Read the model definition and answer for the solid it produces. Units are mm, in the model's axes. A direction names the side the tool comes from. Coordinates: 2 decimals unless noted, no trailing zeros. Write each loop counter-clockwise with the first axis right and the second up, starting at its lowest first coordinate (ties: lowest second). Pieces come first, ordered by that corner, then holes. Notation, with made-up numbers: (-15.75, 87.5) -> (6.25, 87.5) arc R26 ccw to (6.25, 115.5) -> close; hole circle Ø1 at (78.5, 81). An arc over 180 degrees is marked (long way). Answer in a Markdown table with one row per item. Add a question column.
Item 1: Section A-A on y = 16.25 is taken. Write down the section's boundary in (x, z), then the cut area to 3 significant figures.
Item 2: Straight lines are drawn through the part: line 1 (X direction, y = 19, z = -22.1); line 2 (Z direction, x = -20, y = 2.5); line 3 (Z direction, x = 14.5, y = 14). For each, find the intervals that lie inside material, in ascending order. Write a range as from..to.
Item 3: Section D-D on y = 18.75 is taken. Write down the section's boundary in (x, z), then the cut area to 3 significant figures.
Item 4: For a pull along Z with two mould halves and no side action, classify faces 4 (the face through (16, 17, 4)), 5 (the face through (-0.766, 19.788, -20.253)), 6 (the face through (0, 20, -16.1)) as +Z half, -Z half, draft (parallel to the pull), parting line (faces both ways), or undercut.
Item 5: Section C-C on z = -17 is taken. Write down the section's boundary in (x, y).
Item 6: Section B-B on x = 0 is taken. Write down the section's boundary in (y, z).
Item 7: Given pin 1 Ø5 at (x, z) = (-15, -19) entering from -Y; pin 2 Ø3 at (x, y) = (3, 20.5) entering from +Z; pin 3 Ø6 at (x, z) = (-4.5, 1) entering from +Y; pin 4 Ø1.5 at (y, z) = (16.5, -0.5) entering from -X, each flat-ended and moving along its own axis, determine where each tip first touches the part or whether it passes through.
Item 8: Which of the six approach directions +Z, -Z, +X, -X, +Y, -Y give full straight-line access (tool end or side, diameter ignored) to faces 1 (the face through (16, 9, 2.1)), 2 (the face through (0, 17, -22)), 3 (the face through (-9, 9, 4))?
```python
from build123d import *

# Parameters (mm, degrees)
SKETCH1_W      = 45
SKETCH1_H      = 10.2
EXTRUDE1_DEPTH = 2
SKETCH2_W      = 13.5
SKETCH2_H      = 3
SKETCH2_W_2    = 45
EXTRUDE2_DEPTH = 15
SKETCH3_W      = 45
SKETCH3_H      = 4
EXTRUDE3_DEPTH = 23
SKETCH6_W      = 12
SKETCH6_H      = 12
EXTRUDE4_DEPTH = 5.5
SKETCH7_R      = 2
EXTRUDE5_DEPTH = 5.5


with BuildPart() as part:
    # Sketch1 → Extrude1 (new body)
    with BuildSketch(Plane(origin=(0, 0, 0), x_dir=(1, 0, 0), z_dir=(0, 1, 0))):
        Rectangle(SKETCH1_W, SKETCH1_H)
    extrude(amount=EXTRUDE1_DEPTH)

    # Sketch2 → Extrude2 (add)
    with BuildSketch(Plane(origin=(0, 2, 0), x_dir=(1, 0, 0), z_dir=(0, 1, 0))):
        with Locations((-15.75, -3.6)):
            Rectangle(SKETCH2_W, SKETCH2_H)
        with Locations((15.75, -3.6)):
            Rectangle(SKETCH2_W, SKETCH2_H)
        with Locations((0, 3.6)):
            Rectangle(SKETCH2_W_2, SKETCH2_H)
    extrude(amount=EXTRUDE2_DEPTH)

    # Sketch3 → Extrude3 (add)
    with BuildSketch(Plane(origin=(0, 0, -5.1), x_dir=(-1, 0, 0), z_dir=(0, 0, -1))):
        with Locations((0, 15)):
            Rectangle(SKETCH3_W, SKETCH3_H)
    extrude(amount=EXTRUDE3_DEPTH)

    # Sketch6 → Extrude4 (add)
    with BuildSketch(Plane(origin=(0, 17, 0), x_dir=(1, 0, 0), z_dir=(0, 1, 0))):
        with Locations((0, 22.1)):
            Rectangle(SKETCH6_W, SKETCH6_H)
    extrude(amount=EXTRUDE4_DEPTH)

    # Sketch7 → Extrude5 (cut)
    with BuildSketch(Plane(origin=(0, 22.5, 0), x_dir=(1, 0, 0), z_dir=(0, 1, 0))):
        with Locations(Location((0, 22.1, 0), (0, 0, 270))):
            Circle(SKETCH7_R)
    extrude(amount=-EXTRUDE5_DEPTH, mode=Mode.SUBTRACT)


solid = part.part
```
Results below:
| question | item | result |
|---|---|---|
| 1 | outline | (-22.5, -28.1) -> (22.5, -28.1) -> (22.5, -2.1) -> (-22.5, -2.1) -> close; (-22.5, 2.1) -> (-9, 2.1) -> (-9, 5.1) -> (-22.5, 5.1) -> close; (9, 2.1) -> (22.5, 2.1) -> (22.5, 5.1) -> (9, 5.1) -> close |
| 1 | area | 1,250 mm2 |
| 2 | line 1 | x = -6..-2, 2..6 |
| 2 | line 2 | z = -5.1..-2.1, 2.1..5.1 |
| 2 | line 3 | z = -28.1..-2.1, 2.1..5.1 |
| 3 | outline | (-6, -28.1) -> (6, -28.1) -> (6, -16.1) -> (-6, -16.1) -> close; hole circle Ø4 at (0, -22.1) |
| 3 | area | 131 mm2 |
| 4 | face 4 | draft |
| 4 | face 5 | undercut |
| 4 | face 6 | +Z half |
| 5 | outline | (-22.5, 13) -> (22.5, 13) -> (22.5, 17) -> (6, 17) -> (6, 22.5) -> (-6, 22.5) -> (-6, 17) -> (-22.5, 17) -> close |
| 6 | outline | (0, -5.1) -> (13, -5.1) -> (13, -28.1) -> (22.5, -28.1) -> (22.5, -24.1) -> (17, -24.1) -> (17, -20.1) -> (22.5, -20.1) -> (22.5, -16.1) -> (17, -16.1) -> (17, -2.1) -> (2, -2.1) -> (2, 5.1) -> (0, 5.1) -> close |
| 7 | pin 1 | stops at y = 13 |
| 7 | pin 2 | stops at z = -16.1 |
| 7 | pin 3 | stops at y = 2 |
| 7 | pin 4 | passes through |
| 8 | face 1 | +X, -X, +Y |
| 8 | face 2 | +Y |
| 8 | face 3 | +Z, +Y |
